Input: part model. Units: mm. Frame: model coordinates. A direction names the side the tool comes from. Give positions to 0.01 mm unless a question says otherwise; leave off trailing zeros. Loops run counter-clockwise (first coordinate to the right, second up) from the corner with the lowest first, then second, coordinate; pieces in that order, holes last. Notation, with made-up numbers: (8, 42.5) - (51, 42.5) arc R5 ccw to (51, 47.5) - close; hole circle Ø1 at (39.5, 28). An arc over 180 degrees is marked (long way). One line per question, with ' | ' between items. Start each with the question number.
from build123d import *

# Parameters (mm, degrees)
F2_R     = 4
F3_DEPTH = 60


with BuildPart() as f1:
    # F0 (on Top) → F1 (revolve)
    with BuildSketch(Plane.XY):
        Polygon((0, 7.601157), (0, 0), (83.355051, 0), (83.355051, 10.201156), (78.355052, 10.201156), (78.355052, 16.401156), (71.355052, 16.401156), (71.355052, 13.201156), (16.155056, 13.201156), (16.155056, 16.401156), (9.155056, 16.401156), (9.155056, 7.601157), align=None)
    revolve(axis=Axis((41.677526, 0, 0), (-1, 0, 0)))

    # F2 (on face) → F3 (cut)
    with BuildSketch(Plane.YZ.offset(83.355051)):
        Circle(F2_R)
    extrude(amount=-F3_DEPTH, mode=Mode.SUBTRACT)


solid = f1.part
Q1. Section A-A, the plane y = 0. Output: boundary loops of the cut face in (x, z), plus the area to 3 significant figures.
Q2. Draft query along Z for faces 4 (the face through (53.775, -0.867, -3.905)), 5 (the face through (0, 0, 0)), 6 (the face through (80.82, 9.73, -3.06)). Return one class per face: +Z half, -Z half, draft (parallel to the pull), parting line (faces both ways), or undercut.
Q3. Section D-D, the plane z = 9. Output: boundary loops of the cut face in (x, y).
Q4. Line query: L1, parallel to Z at x = 62, y = 0; L2, parallel to X at y = -7, z = 11.5; L3, parallel to X at y = -7.5, z = -10. Output: solid intervals per line, ascending. Write a range as from..to.
Q5. Section C-C, the plane x = 66. Output: boundary loops of the cut face in (y, z), plus the area to 3 significant figures.
Q6. First-contact query: pin 1 (6 mm diameter, centred on x = 28, z = 4.5, fed in from +Y); pin 2 (3 mm diameter, centred on x = 72, z = 2, fed in from +Y); pin 3 (10 mm diameter, centred on x = 21.5, y = 0, fed in from -Z). Flat tips, straight axial feed; report the tip coordinate or a pass-through.
Q7. Access query for faces 1 (the face through (4.51, 7.25, -2.28)), 2 (the face through (78.355, 8, 7)), 3 (the face through (16.155, -1.1, -13.4)). Directions: +Z, -Z, +X, -X, +Y, -Y. A direction counts if a zero-diameter tool reaches every point of the face in a straight line with its end or side. Return the directions, or none.
Solved:
1) outline: (0, -7.6) - (9.16, -7.6) - (9.16, -16.4) - (16.16, -16.4) - (16.16, -13.2) - (71.36, -13.2) - (71.36, -16.4) - (78.36, -16.4) - (78.36, -10.2) - (83.36, -10.2) - (83.36, -4) - (23.36, -4) - (23.36, 4) - (83.36, 4) - (83.36, 10.2) - (78.36, 10.2) - (78.36, 16.4) - (71.36, 16.4) - (71.36, 13.2) - (16.16, 13.2) - (16.16, 16.4) - (9.16, 16.4) - (9.16, 7.6) - (0, 7.6) - close | area: 1,680 mm²
2) face 4: undercut | face 5: draft | face 6: parting line
3) outline: (9.16, -13.71) - (16.16, -13.71) - (16.16, -9.66) - (71.36, -9.66) - (71.36, -13.71) - (78.36, -13.71) - (78.36, -4.8) - (83.36, -4.8) - (83.36, 4.8) - (78.36, 4.8) - (78.36, 13.71) - (71.36, 13.71) - (71.36, 9.66) - (16.16, 9.66) - (16.16, 13.71) - (9.16, 13.71) - close
4) L1: z = -13.2..-4, 4..13.2 | L2: x = 9.16..16.16, 71.36..78.36 | L3: x = 9.16..78.36
5) outline: circle Ø26.4 at (0, 0); hole circle Ø8 at (0, 0) | area: 497 mm²
6) pin 1: stops at y = 13.12 | pin 2: stops at y = 16.39 | pin 3: stops at z = -13.2
7) face 1: -X | face 2: +X | face 3: none
